Study the drawing (mm; zero at the part's minimum x, y, z) and answer. Give positions to 0.01 mm unless a question says otherwise; leave off trailing zeros. Write each loop counter-clockwise with the first axis right and the second up, starting at its lowest first coordinate (ties: lowest second). Pieces come first, ordered by that corner, then holes. Notation, with made-up numbers: (44, -7) - (80, -7) arc R17 ccw to (80, 3) - close; hole circle Ø7 at (-17, -35.75). An arc over 180 degrees is marked (long way). Answer as CSV lines item,"result".
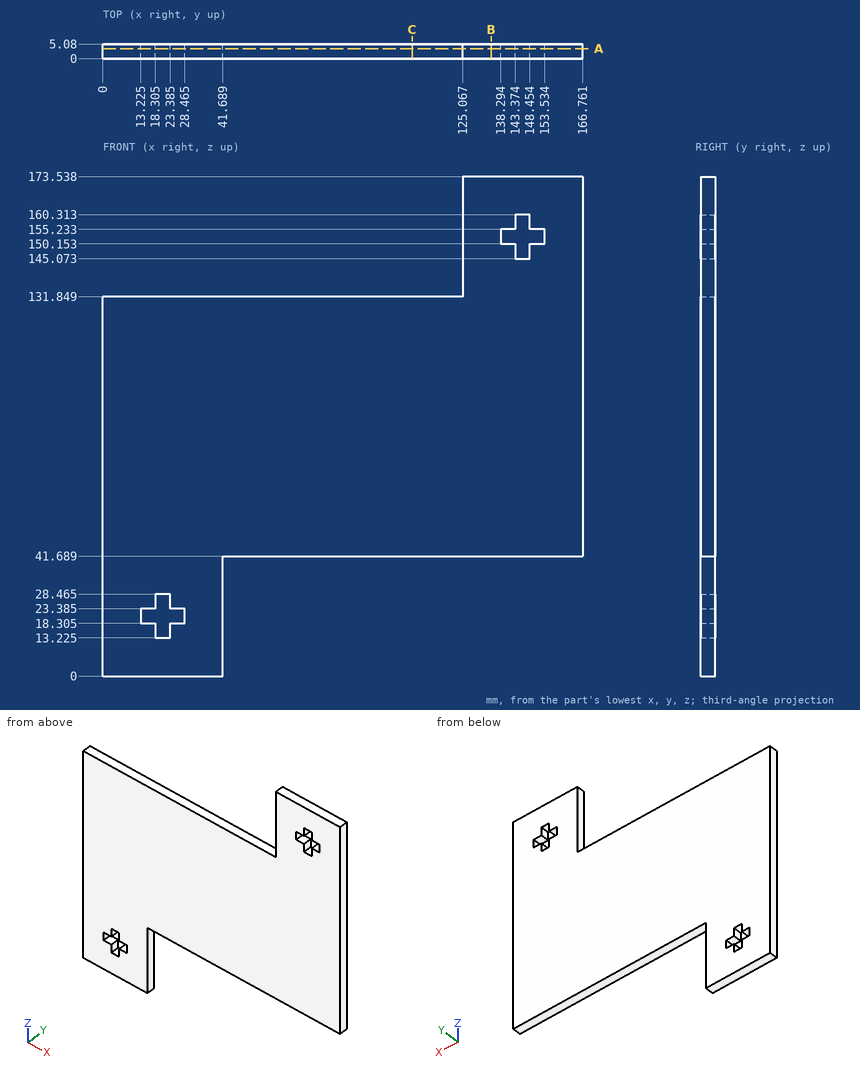
(1) Find the intervals of material crossed by L1, parallel to Z at x = 15, y = 3.4 (1 decimal); L2, parallel to Z at x = 152.5, y = 2.5; L3, parallel to Z at x = 79.5, y = 4.7, in increasing order.
Worked out:
L1,"z = 0 to 18.3, 23.4 to 131.8"
L2,"z = 41.69 to 150.15, 155.23 to 173.54"
L3,"z = 41.69 to 131.85"
(2) A cutting plane is placed at B-B (x = 135). Write down the section's boundary in (y, z), and give its area (3 significant figures).
Worked out:
outline,"(0, 41.69) - (5.08, 41.69) - (5.08, 173.54) - (0, 173.54) - close"
area,"670 mm^2"
(3) A cutting plane is placed at C-C (x = 107.5). Write down the section's boundary in (y, z), and give its area (3 significant figures).
Worked out:
outline,"(0, 41.69) - (5.08, 41.69) - (5.08, 131.85) - (0, 131.85) - close"
area,"458 mm^2"
(4) A cutting plane is placed at A-A (y = 3.5). Count the separate pieces of the cut face and the enclosed holes in it, and give its area (3 significant figures).
Worked out:
separate pieces,"1"
enclosed holes,"2"
area,"18,300 mm^2"
(5) Each of these flat-tipped pins is pushed along its axis until it touches: P1, Ø1.5, axis at x = 21.5, y = 2.5, coming from the -Z side; P2, Ø1.5, axis at x = 152, y = 2.5, coming from the -Z side; P3, Ø2.5, axis at y = 3, z = 21.5, coming from the +X side; P4, Ø3, axis at x = 121.5, y = 3.5, coming from the +Z side. Where does it stop, or does it pass through?
Worked out:
P1,"stops at z = 0"
P2,"stops at z = 41.69"
P3,"stops at x = 41.69"
P4,"stops at z = 131.85"
